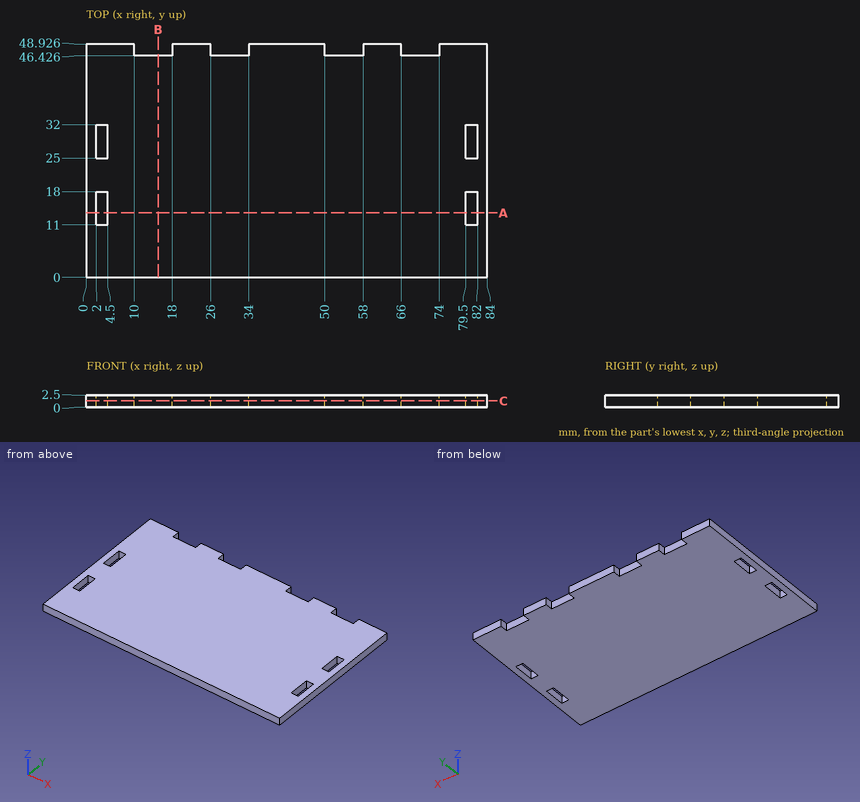
Could you check a few things on this drawing? It's one solid part, dimensions in mm from its lowest x, y, z. Give positions to 0.01 mm unless a question says otherwise; leave off trailing zeros. Loops run counter-clockwise (first coordinate to the right, second up) from the corner with the lowest first, then second, coordinate; pieces in that order, holes last. Notation, with made-up numbers: M 4.5,-5 L 38.5,-5 A18 ccw 38.5,3 Z; hole C 1,14 d9. An arc over 180 degrees is marked long. Return JSON: item names as keys, results as strings.
Item 1: Please list where these lines run through material, in increasing order: line 1 (X direction, y = 29, z = 1.85); line 2 (Y direction, x = 10.5, z = 1.2).
A:
{"line 1": "x = 0 to 2, 4.5 to 79.5, 82 to 84", "line 2": "y = 0 to 46.43"}
Item 2: Imagine slicing it at B-B on x = 15. List the corners of the cut face in (y, z) for me, then the cut area to 3 significant figures.
A:
{"outline": "M 0,0 L 46.43,0 L 46.43,2.5 L 0,2.5 Z", "area": "116 mm^2"}
Item 3: Imagine slicing it at A-A on y = 13.5. List the corners of the cut face in (x, z) for me.
A:
{"outline": "M 0,0 L 2,0 L 2,2.5 L 0,2.5 Z; M 4.5,0 L 79.5,0 L 79.5,2.5 L 4.5,2.5 Z; M 82,0 L 84,0 L 84,2.5 L 82,2.5 Z"}
Item 4: Imagine slicing it at C-C on z = 1.35. State how many separate pieces and enclosed holes the cut face has, then the cut area to 3 significant figures.
A:
{"separate pieces": "1", "enclosed holes": "4", "area": "3,960 mm^2"}
Item 5: I'm going to push a flat-ended pin straight in: pin 1 Ø0.8 at (x, z) = (52.5, 1) entering from +Y. Where does the tip first touch, or does it pass through?
A:
{"pin 1": "stops at y = 46.43"}
